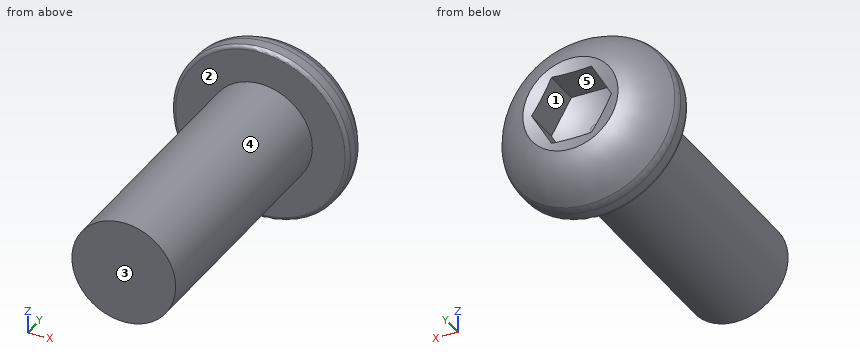
from build123d import *

# Parameters (mm, degrees)
FILLET1_R           = 0.2
FILLET2_R           = 1
SKETCH2_R           = 3
BOSS_EXTRUDE1_DEPTH = 15
CUT_EXTRUDE1_DEPTH  = 2.3


with BuildPart() as part:
    # Sketch1 → Revolve1 (revolve)
    with BuildSketch(Plane.XY):
        with BuildLine():
            Line((0, 0), (5.1, 0))
            Line((5.1, 0), (5.1, 1))
            ThreePointArc((5.1, 1), (4.1560785, 2.346833852), (2.75, 3.2))
            Line((2.75, 3.2), (0, 3.2))
            Line((0, 3.2), (0, 0))
        make_face()
    revolve(axis=Axis((0, 55, 0), (0, -1, 0)))

    # Fillet1
    fillet1_edges = [part.edges().sort_by_distance(p)[0] for p in [
        (-5.1, 0, 0),
    ]]
    fillet(fillet1_edges, radius=FILLET1_R)

    # Fillet2
    fillet2_edges = [part.edges().sort_by_distance(p)[0] for p in [
        (-5.1, 1, 0),
    ]]
    fillet(fillet2_edges, radius=FILLET2_R)

    # Sketch2 → Boss-Extrude1 (add)
    with BuildSketch(Plane.XZ):
        Circle(SKETCH2_R)
    extrude(amount=BOSS_EXTRUDE1_DEPTH)

    # Sketch6 → Revolve2 (revolve)
    with BuildSketch(Plane.XY):
        Polygon((0, 0), (0, 3.2), (2.75, 3.2), (4.9, 0), align=None)
    revolve(axis=Axis((0, 55, 0), (0, -1, 0)))

    # Sketch7 → Cut-Extrude1 (cut)
    with BuildSketch(Plane(origin=(0, 3.2, 0), x_dir=(1, 0, 0), z_dir=(0, 1, 0))):
        Polygon((1.154700538, -2), (2.309401077, 0), (1.154700538, 2), (-1.154700538, 2), (-2.309401077, 0), (-1.154700538, -2), align=None)
    extrude(amount=-CUT_EXTRUDE1_DEPTH, mode=Mode.SUBTRACT)

    # Sketch8 → Cut-Revolve1 (revolve, cut)
    with BuildSketch(Plane.XY):
        with BuildLine():
            Line((0, 0.9), (0, 0.5))
            Line((0, 0.5), (0.25, 0.5))
            ThreePointArc((0.25, 0.5), (1.298943849, 0.600925763), (2.309401077, 0.9))
            Line((2.309401077, 0.9), (0, 0.9))
        make_face()
    revolve(axis=Axis((0, 55, 0), (0, -1, 0)), mode=Mode.SUBTRACT)

    # Sketch9 → Cut-Revolve2 (revolve, cut)
    with BuildSketch(Plane.XY):
        with BuildLine():
            ThreePointArc((0, 2.814442262), (1.388448304, 2.911300775), (2.75, 3.2))
            Line((2.75, 3.2), (0, 3.2))
            Line((0, 3.2), (0, 2.814442262))
        make_face()
    revolve(axis=Axis((0, 55, 0), (0, -1, 0)), mode=Mode.SUBTRACT)


solid = part.part
Can you work these out from the model? Positions are in its coordinate system, mm. Face numbers are marked on the shaded views. A direction names the side the tool comes from. Round coordinates to 2 decimals unless told otherwise and drop trailing zeros. Write each loop counter-clockwise with the first axis right and the second up, starting at its lowest first coordinate (ties: lowest second). Pieces come first, ordered by that corner, then holes. Notation, with made-up numbers: (66.25, 84.25) -> (78.25, 84.25) arc R10 ccw to (78.25, 97.25) -> close; hole circle Ø10 at (86, -19). An arc over 180 degrees is marked (long way). Use one line per item in the form item = value. Start each with the question number.
Q1. Imagine slicing it at A-A (y = -10.25). Please give me the cut outline in (x, z), then the cut area to 3 significant figures.
Q2. If I drill on probe 1 along Z at (x, y) = (0, 2.5); probe 2 along Y at (x, z) = (2, -3); probe 3 along Z at (x, y) = (-2, 1), over which ranges is the centre line in solid material (lowest first)? Write a range as [from, to].
Q3. Which directions (+Z, -Z, +X, -X, +Y, -Y) give clear straight access to the entire face, cutting with the end or side of a thin tool? Please do the marked faces 1 and 2.
Q4. I'm going to push flat-ended pins straight in: P1, Ø2, axis at x = -1.5, y = -1.5, coming from the -Z side; P2, Ø1.7, axis at x = -0.5, y = 2.5, coming from the -Z side; P3, Ø2, axis at y = -10.5, z = 0, coming from the -X side. Where does each tip first touch, or does it pass through?
Q5. We'd pull the mould along X, two halves only. Please class the marked faces 3, 4 and 5: +X half, -X half, draft (parallel to the pull), parting line (faces both ways), or undercut.
Worked out:
q1.outline = circle Ø6 at (0, 0)
q1.area = 28.3 mm^2
q2.probe_1 = [-3.98, -2], [2, 3.98]
q2.probe_2 = [0, 2.78]
q2.probe_3 = [-4.66, -0.54], [0.54, 4.66]
q3.face_1 = +Y
q3.face_2 = -Y
q4.P1 = -2.96
q4.P2 = -4.73
q4.P3 = -3
q5.face_3 = draft
q5.face_4 = parting line
q5.face_5 = undercut
